```python
from build123d import *

# Parameters (mm, degrees)
SKETCH1_R           = 30
SKETCH1_R_2         = 7
BOSS_EXTRUDE1_DEPTH = 10
FILLET1_R           = 10
FILLET2_R           = 20
CUT_EXTRUDE1_DEPTH  = 21


with BuildPart() as part:
    # Sketch1 → Boss-Extrude1 (new body, symmetric)
    with BuildSketch(Plane(origin=(0, 0, 0), x_dir=(1, 0, 0), z_dir=(0, 1, 0))):
        with BuildLine():
            Line((9.080898408, 13.654134499), (-90.777819418, 30.604008061))
            ThreePointArc((-90.777819418, 30.604008061), (-156.75035362, 4.883640056), (-90.777819418, -20.836727949))
            Line((-90.777819418, -20.836727949), (9.080898408, -3.886854388))
            ThreePointArc((9.080898408, -3.886854388), (36.24964638, 4.883640056), (9.080898408, 13.654134499))
        make_face()
        with Locations((-118.75035362, 4.883640056)):
            Circle(SKETCH1_R, mode=Mode.SUBTRACT)
        with Locations((21.24964638, 4.883640056)):
            Circle(SKETCH1_R_2, mode=Mode.SUBTRACT)
    extrude(amount=BOSS_EXTRUDE1_DEPTH, both=True)

    # Fillet1
    fillet1_edges = [part.edges().sort_by_distance(p)[0] for p in [
        (9.080898408, 0, -13.654134499),
        (9.080898408, 0, 3.886854388),
    ]]
    fillet(fillet1_edges, radius=FILLET1_R)

    # Fillet2
    fillet2_edges = [part.edges().sort_by_distance(p)[0] for p in [
        (-90.777819418, 0, 20.836727949),
        (-90.777819418, 0, -30.604008061),
    ]]
    fillet(fillet2_edges, radius=FILLET2_R)

    # Sketch2 → Cut-Extrude1 (cut, through all)
    with BuildSketch(Plane(origin=(0, 10, 0), x_dir=(1, 0, 0), z_dir=(0, 1, 0))):
        with BuildLine():
            Line((-76.385663344, 22.582436294), (1.373906039, 9.383640056))
            ThreePointArc((1.373906039, 9.383640056), (5.873906039, 4.883640056), (1.373906039, 0.383640056))
            Line((1.373906039, 0.383640056), (-76.385663344, -12.815156183))
            ThreePointArc((-76.385663344, -12.815156183), (-82.031183012, -11.100966392), (-82.113079878, -5.201506089))
            ThreePointArc((-82.113079878, -5.201506089), (-80.75035362, 4.883640056), (-82.113079878, 14.968786201))
            ThreePointArc((-82.113079878, 14.968786201), (-82.031183012, 20.868246504), (-76.385663344, 22.582436294))
        make_face()
    extrude(amount=-CUT_EXTRUDE1_DEPTH, mode=Mode.SUBTRACT)


solid = part.part
```
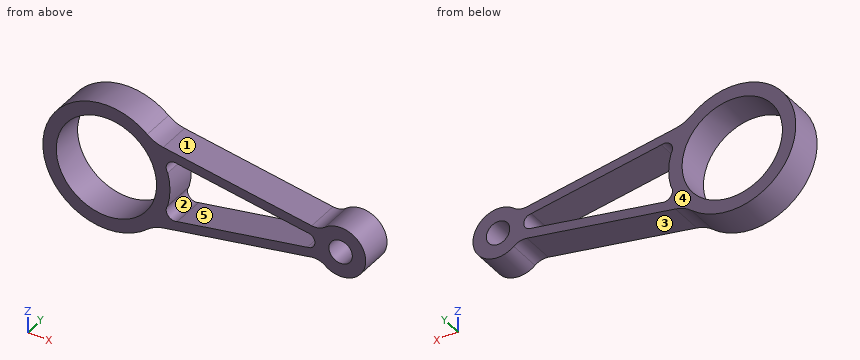
Part model, mm, in its own coordinate system. Face numbers are marked on the shaded views. A direction names the side the tool comes from. Give positions to 0.01 mm unless a question says otherwise; leave off trailing zeros. Write each loop counter-clockwise with the first axis right and the second up, starting at its lowest first coordinate (ties: lowest second). Pieces come first, ordered by that corner, then holes. Notation, with made-up numbers: (52, -18) -> (99, -18) arc R23 cw to (99, -10) -> close; hole circle Ø3 at (37.25, 18). An arc over 180 degrees is marked (long way). Put each result on its own line as item: value. Start each with the question number.
Item 1: Cut at D-D (z = -2.5). List the corners of the cut face in (x, y).
Item 2: Cut at C-C (y = -4.5). List the corners of the cut face in (x, z).
Item 3: Which spindle directions (+Z, -Z, +X, -X, +Y, -Y) get a long thin tool onto all of the face, cutting with end or side? Do the marked faces 4 and 5. Say none if no direction does.
Item 4: Pull direction Z, two halves, no side cores. Call the marked faces 1, 2 and 3: pulls with the +Z half, pulls with the -Z half, needs draft (parallel to the pull), parting line crosses it, or undercut.
Item 5: Pin check, flat tips, straight feed: pin 1 Ø2 at (x, y) = (12.5, -6) entering from +Z; pin 2 Ø8 at (x, y) = (-51, 5) entering from +Z; pin 3 Ø6 at (y, z) = (-2, -21) entering from +X. Stop position of each tip, or through.
Item 6: Cut at A-A (z = 16.5). List the corners of the cut face in (x, y).
Item 7: Cut at B-B (x = -54). List the corners of the cut face in (y, z).
Item 8: Wall check: L1, parallel to X at y = -5.5, z = -5.5; L2, parallel to Z at x = -42, y = 3.25; L3, parallel to Z at x = -91, y = -0.5. Give the ranges that are in metal, low to high. Write a range as [from, to].
Answer list:
1. outline: (-156.68, -10) -> (-148.66, -10) -> (-148.66, 10) -> (-156.68, 10) -> close; (-88.85, -10) -> (-80.83, -10) -> (-80.83, 10) -> (-88.85, 10) -> close; (5.19, -10) -> (14.67, -10) -> (14.67, 10) -> (5.19, 10) -> close; (27.83, -10) -> (36.06, -10) -> (36.06, 10) -> (27.83, 10) -> close
2. outline: (-94.32, -33.99) arc R20 cw to (-84.81, -29.59) -> (3.94, -14.53) arc R10 cw to (11.87, -16.59) arc R15 ccw (long way) to (11.87, 6.82) arc R10 cw to (3.94, 4.76) -> (-84.81, 19.82) arc R20 cw to (-94.32, 24.22) arc R38 ccw (long way) to start; hole circle Ø60 at (-118.75, -4.88); hole (-82.11, -14.97) arc R5 ccw to (-76.39, -22.58) -> (1.37, -9.38) arc R4.5 ccw to (1.37, -0.38) -> (-76.39, 12.82) arc R5 ccw to (-82.11, 5.2) arc R38 cw to start; hole circle Ø14 at (21.25, -4.88)
3. face 4: +Z, -Z, +X, -X, +Y
3. face 5: +Y, -Y
4. face 1: pulls with the +Z half
4. face 2: undercut
4. face 3: pulls with the -Z half
5. pin 1: stops at z = 7.96
5. pin 2: stops at z = 14.76
5. pin 3: stops at x = 28.53
6. outline: (-150.16, -10) -> (-139.79, -10) -> (-139.79, 10) -> (-150.16, 10) -> close; (-97.71, -10) -> (-65.23, -10) -> (-65.23, 10) -> (-97.71, 10) -> close
7. outline: (-10, -24.36) -> (10, -24.36) -> (10, -18.78) -> (-10, -18.78) -> close; (-10, 9.02) -> (10, 9.02) -> (10, 14.59) -> (-10, 14.59) -> close
8. L1: x = [-156.75, -148.74], [-88.76, -80.76], [5.83, 14.28], [28.22, 36.24]
8. L2: z = [-22.32, -16.75], [6.98, 12.56]
8. L3: z = [-31.73, -16.28], [6.51, 21.96]
